Design review of the part shown in the three views and the two pictorial views. Dimensions are in mm from the part's minimum x, y and z. A direction names the side the tool comes from. Give positions to 0.01 mm unless a question says otherwise; leave off trailing zeros. Loops run counter-clockwise (first coordinate to the right, second up) from the corner with the lowest first, then second, coordinate; pieces in that order, holes last.
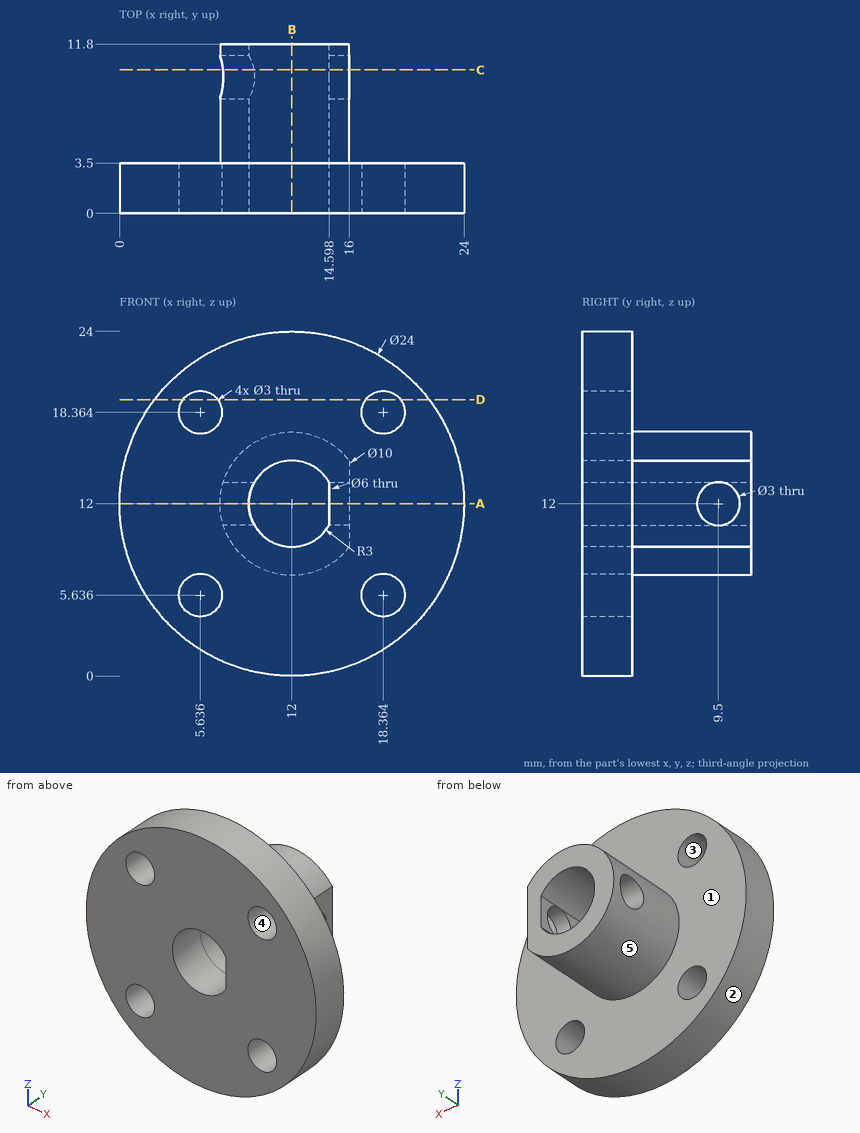
Q1. Take a section at C-C (y = 10). Give the boundary of the cut face in (x, z), plus the area to 3 significant figures.
Results:
outline: (7.2, 10.59) arc R5 ccw to (16, 9) - (16, 10.59) - (14.6, 10.59) - (14.6, 10.5) arc R3 cw to (9.35, 10.59) - close; (7.2, 13.41) - (9.35, 13.41) arc R3 cw to (14.6, 13.5) - (14.6, 13.41) - (16, 13.41) - (16, 15) arc R5 ccw to start
area: 37.2 mm2
Q2. Draft analysis for pull direction X (two halves, no side actions). For the marked faces 1, 2 and 3, state which applies: pulls with the +X half, pulls with the -X half, needs draft (parallel to the pull), parting line crosses it, or undercut.
Results:
face 1: needs draft
face 2: parting line crosses it
face 3: undercut
Q3. Take a section at B-B (x = 12). Give the boundary of the cut face in (y, z), plus the area to 3 significant figures.
Results:
outline: (0, 0) - (3.5, 0) - (3.5, 7) - (11.8, 7) - (11.8, 9) - (0, 9) - close; (0, 15) - (11.8, 15) - (11.8, 17) - (3.5, 17) - (3.5, 24) - (0, 24) - close
area: 96.2 mm2
Q4. Take a section at A-A (z = 12). Give the boundary of the cut face in (x, y).
Results:
outline: (0, 0) - (9, 0) - (9, 8) - (7, 8) - (7, 3.5) - (0, 3.5) - close; (7, 11) - (9, 11) - (9, 11.8) - (7, 11.8) - close; (14.6, 0) - (24, 0) - (24, 3.5) - (16, 3.5) - (16, 8) - (14.6, 8) - close; (14.6, 11) - (16, 11) - (16, 11.8) - (14.6, 11.8) - close
Q5. Take a section at D-D (z = 19.25). Give the boundary of the cut face in (x, y), plus the area to 3 significant figures.
Results:
outline: (2.44, 0) - (4.43, 0) - (4.43, 3.5) - (2.44, 3.5) - close; (6.85, 0) - (17.15, 0) - (17.15, 3.5) - (6.85, 3.5) - close; (19.57, 0) - (21.56, 0) - (21.56, 3.5) - (19.57, 3.5) - close
area: 50.0 mm2
Q6. Tool access review of the marked faces 4 and 5: name each direction out of +Z, -Z, +X, -X, +Y, -Y from which nothing blocks a thin tool from reaching the whole face with its end or side.
Results:
face 4: +Y, -Y
face 5: +Y
Q7. Wall thickness on line 1 (Z direction, x = 18.5, y = 1); line 2 (Z direction, x = 12, y = 9.25); line 3 (Y direction, x = 7.5, z = 22.5): over which ranges is each line inside the solid? List them lowest first.
Results:
line 1: z = 1.91 to 4.14, 7.13 to 16.87, 19.86 to 22.09
line 2: z = 7 to 9, 15 to 17
line 3: y = 0 to 3.5
Q8. Insertion check: pin 1 (3.5 mm diameter, centred on y = 9.5, z = 12, fed in from -X); pin 2 (1.5 mm diameter, centred on y = 8, z = 15, fed in from -X) (3 decimals); pin 3 (3 mm diameter, centred on x = 3, y = 5.5, fed in from +Z); pin 4 (4 mm diameter, centred on y = 9.5, z = 12, fed in from +X). Each pin has a flat end and moves straight along its axis. Give the tip position at first contact, or say it passes through.
Results:
pin 1: stops at x = 7
pin 2: stops at x = 7.535
pin 3: passes through
pin 4: stops at x = 16
